```python
from build123d import *

# Parameters (mm, degrees)
SKETCH1_W               = 276.225
SKETCH1_H               = 152.4
BULK_EXTRUDE_DEPTH      = 136.525
SKETCH1_13_W            = 273.177
SKETCH1_13_H            = 149.352
SKETCH1_13_W_2          = 245.745
SKETCH1_13_H_2          = 1.524
INNER_SHELL_CUT_DEPTH   = 120.65
SKETCH1_14_W            = 245.745
SKETCH1_14_H            = 1.524
TOP_WALL_EXTRUDE_DEPTH  = 15.24
TOP_START               = -15.24
SKETCH1_15_W            = 273.177
SKETCH1_15_H            = 149.352
TOP_FLOOR_EXTRUDE_DEPTH = 1.524
SKETCH5_R               = 1.651
HINGE_EXTRUDE_DEPTH     = 82.55
SKETCH7_W               = 25.4635
SKETCH7_H               = 19.05
RAILS_EXTRUDE_DEPTH     = 125.476


with BuildPart() as part:
    # Sketch1 → Bulk-Extrude (new body)
    with BuildSketch(Plane(origin=(0, 0, 0), x_dir=(1, 0, 0), z_dir=(0, 1, 0))):
        with Locations((136.5885, 74.676)):
            Rectangle(SKETCH1_W, SKETCH1_H)
    extrude(amount=-BULK_EXTRUDE_DEPTH)

    # Sketch1<13> → Inner Shell-Cut (cut)
    with BuildSketch(Plane(origin=(0, 0, 0), x_dir=(1, 0, 0), z_dir=(0, 1, 0))):
        with Locations((136.5885, 74.676)):
            Rectangle(SKETCH1_13_W, SKETCH1_13_H)
        with Locations((136.5885, -0.762)):
            Rectangle(SKETCH1_13_W_2, SKETCH1_13_H_2)
    extrude(amount=-INNER_SHELL_CUT_DEPTH, mode=Mode.SUBTRACT)

    # Sketch1<14> → Top Wall-Extrude (add)
    with BuildSketch(Plane(origin=(0, 0, 0), x_dir=(1, 0, 0), z_dir=(0, 1, 0))):
        with Locations((136.5885, -0.762)):
            Rectangle(SKETCH1_14_W, SKETCH1_14_H)
    extrude(amount=-TOP_WALL_EXTRUDE_DEPTH)

    # Sketch1<15> → Top Floor-Extrude (add)
    with BuildSketch(Plane(origin=(0, 0, 0), x_dir=(1, 0, 0), z_dir=(0, 1, 0)).offset(TOP_START)):
        with Locations((136.5885, 74.676)):
            Rectangle(SKETCH1_15_W, SKETCH1_15_H)
    extrude(amount=TOP_FLOOR_EXTRUDE_DEPTH)

    # Sketch5 → Hinge-Extrude (add)
    with BuildSketch(Plane(origin=(274.701, 0, 0), x_dir=(0, 0, -1), z_dir=(1, 0, 0))):
        with BuildLine():
            Line((150.876, 0), (150.876, -3.175))
            Line((150.876, -3.175), (154.051, -3.175))
            ThreePointArc((154.051, -3.175), (156.29606403, 2.24506403), (150.876, 0))
        make_face()
        with Locations((154.051, 0)):
            Circle(SKETCH5_R, mode=Mode.SUBTRACT)
    hinge_extrude = extrude(amount=-HINGE_EXTRUDE_DEPTH)

    # Mirror1: Hinge-Extrude across plane
    add(hinge_extrude.mirror(Plane(origin=(136.5885, 0, 0), x_dir=(0, 0, 1), z_dir=(1, 0, 0))))

    # Sketch7 → Rails-Extrude (add)
    with BuildSketch(Plane.XY.offset(-149.352)):
        with Locations((12.73175, -43.815)):
            Rectangle(SKETCH7_W, SKETCH7_H)
        with Locations((260.44525, -43.815)):
            Rectangle(SKETCH7_W, SKETCH7_H)
        with Locations((12.73175, -94.615)):
            Rectangle(SKETCH7_W, SKETCH7_H)
        with Locations((260.44525, -94.615)):
            Rectangle(SKETCH7_W, SKETCH7_H)
    extrude(amount=RAILS_EXTRUDE_DEPTH)


solid = part.part
```
Can you work these out from the model? Positions are in its coordinate system, mm. A direction names the side the tool comes from. Give positions to 0.01 mm unless a question says otherwise; leave off trailing zeros. Order: outer loops, then holes, each group sorted by start corner. A loop starts at its lowest first (then second) coordinate and runs counter-clockwise, first axis right, second up. Notation, with made-up numbers: M 30.25,-10 L 36.25,-10 A16 ccw 36.25,16 Z; hole C -11,79.5 d10. An arc over 180 degrees is marked long. Write item = value, one per line. Start each with the question number.
Q1. Suppose I cut it at A-A (x = 59.5). Write out the boundary of the cut face in (y, z) (3 decimals), plus the area to 3 significant figures.
Q2. For faces 3 (the flat face through (13, -53.34, -87)), 4 (the flat face through (247.713, -95, -87)), 5 (the flat face through (135, -7, -149.352)), 6 (the flat face through (81.026, -1.4, -152.6)), which set-ups out of +Z, -Z, +X, -X, +Y, -Y let a thin tool reach every point of the face, with its end or its side?
Q3. Will these pins go through, and if not, where does the flat tip stop? pin 1 Ø4 at (x, z) = (167.5, -114.5) entering from +Y; pin 2 Ø8 at (x, y) = (120.5, -115.5) entering from +Z; pin 3 Ø7 at (x, y) = (265, -62) entering from -Z; pin 4 Ø3 at (y, z) = (-1, -155) entering from +X.
Q4. We'd pull the mould along Z, two halves only. Please class faces 1 (the flat face through (266, -67, 0)), 2 (the flat face through (25.464, -95, -87)): pulls with the +Z half, pulls with the -Z half, needs draft (parallel to the pull), parting line crosses it, or undercut.
Q5. Suppose I cut it at C-C (x = 135.5). Write out the boundary of the cut face in (y, z) (3 decimals), plus the area to 3 significant figures.
Q6. I need wall thicknesses on probe 1 along Y at (x, z) = (12.5, -86) (3 decimals); probe 2 along Y at (x, z) = (199.5, -70) (3 decimals); probe 3 along X at (y, z) = (-99, -130.5). Which ranges of each line are inside material? Lowest first, please. Write a range as [from, to].
Check result:
q1.outline = M -136.525,-150.876 L -3.175,-150.876 L -3.175,-154.051 A3.175 ccw long 0,-150.876 L 0,-149.352 L -13.716,-149.352 L -13.716,0 L 0,0 L 0,1.524 L -15.24,1.524 L -15.24,-149.352 L -120.65,-149.352 L -120.65,1.524 L -136.525,1.524 Z; hole C 0,-154.051 d3.302
q1.area = 2,880 mm2
q2.face_3 = none
q2.face_4 = +Z
q2.face_5 = +Y
q2.face_6 = -Z, +Y, -Y
q3.pin_1 = -13.72
q3.pin_2 = -149.35
q3.pin_3 = -150.88
q3.pin_4 = 274.7
q4.face_1 = undercut
q4.face_2 = needs draft
q5.outline = M -136.525,-150.876 L 0,-150.876 L 0,-149.352 L -13.716,-149.352 L -13.716,0 L 0,0 L 0,1.524 L -15.24,1.524 L -15.24,-149.352 L -120.65,-149.352 L -120.65,1.524 L -136.525,1.524 Z
q5.area = 2,850 mm2
q6.probe_1 = [-136.525, -120.65], [-104.14, -85.09], [-53.34, -34.29], [-15.24, -13.716]
q6.probe_2 = [-136.525, -120.65], [-15.24, -13.716]
q6.probe_3 = [-1.52, 25.46], [247.71, 274.7]
